Autodesk Inventor part; units mm, degrees
ref_plane "YZ Plane" through (0, 0, 0) normal (1, 0, 0) x (0, 1, 0)
ref_plane "XZ Plane" through (0, 0, 0) normal (0, 1, 0) x (-1, 0, 0)
ref_plane "XY Plane" through (0, 0, 0) normal (0, 0, 1) x (1, 0, 0)
sketch "Sketch1" plane through (0, 0, 0) normal (0, 1, 0) x (-1, 0, 0)
  line L0 (9.8554, 3.698) -> (9.8554, -5.5599)
  line L1 (0, 0) -> (-5.6892, 0)
  circle A0 centre (-2.8446, 0) radius 1.5875
  circle A1 centre (-2.8446, -12.7) radius 1.5875
  circle A2 centre (-2.8446, -25.4) radius 1.5875
  circle A3 centre (-2.8446, -38.1) radius 1.5875
  line L2 (0, 12.7) -> (-5.6892, 12.7)
  circle A4 centre (-2.8446, 12.7) radius 1.5875
  line L3 (0, 25.4) -> (-5.6892, 25.4)
  circle A5 centre (-2.8446, 25.4) radius 1.5875
  line L4 (0, 38.1) -> (-5.6892, 38.1)
  circle A6 centre (-2.8446, 38.1) radius 1.5875
  line L5 (-12.7, 0) -> (-18.3892, 0)
  circle A7 centre (-15.5446, 0) radius 1.5875
  line L6 (-25.4, 0) -> (-31.0892, 0)
  circle A8 centre (-28.2446, 0) radius 1.5875
  line L7 (-38.1, 0) -> (-43.7892, 0)
  circle A9 centre (-40.9446, 0) radius 1.5875
  line L8 (-50.8, 0) -> (-56.4892, 0)
  circle A10 centre (-53.6446, 0) radius 1.5875
  line L9 (-63.5, 0) -> (-69.1892, 0)
  circle A11 centre (-66.3446, 0) radius 1.5875
  line L10 (9.8554, 3.698) -> (9.8554, 44.45)
  line L11 (9.8554, 44.45) -> (-15.5446, 44.45)
  line L12 (-15.5446, 44.45) -> (-15.5446, 12.7)
  line L13 (-15.5446, 12.7) -> (-72.6946, 12.7)
  line L14 (-72.6946, 12.7) -> (-72.6946, -12.7)
  line L15 (-72.6946, -12.7) -> (-15.5446, -12.7)
  line L16 (-15.5446, -12.7) -> (-15.5446, -44.45)
  line L17 (-15.5446, -44.45) -> (9.8554, -44.45)
  line L18 (9.8554, -5.5599) -> (9.8554, -44.45)
  line L19 (-12.3696, 44.45) -> (-15.5446, 41.275)
  line L20 (6.6804, 44.45) -> (9.8554, 41.275)
  line L21 (9.8554, -41.275) -> (6.6804, -44.45)
  line L22 (-15.5446, -41.275) -> (-12.3696, -44.45)
  line L23 (-69.5196, 12.7) -> (-72.6946, 9.525)
  line L24 (-72.6946, -9.525) -> (-69.5196, -12.7)
  point P0 (-72.6946, 0)
  point P1 (-66.3446, 0)
  dimension "d0" = 3.175
  dimension "d1" = 12.7
  dimension "d4" = 12.7
  dimension "d11" = 12.7
  dimension "d18" = 12.7
  dimension "d23" = 25.4
  dimension "d24" = 6.35
  dimension "d25" = 12.7
  dimension "d26" = 6.35
  dimension "d27" = 25.4
extrude "Extrusion1" add sketch "Sketch1" along normal blind 3.175 contours L0 L18 L21 L17 L22 L16 L15 L24 L14 L23 L13 L12 L19 L11 L20 L10
properties part number "T-Bracket"
Part model, mm, in its own coordinate system. A direction names the side the tool comes from. Round coordinates to 2 decimals unless told otherwise and drop trailing zeros. Write each loop counter-clockwise with the first axis right and the second up, starting at its lowest first coordinate (ties: lowest second). Pieces come first, ordered by that corner, then holes.
Item 1: Drop flat-ended pins along their axis: pin 1 Ø1.9 at (x, z) = (2.84, 25.4) entering from +Y; pin 2 Ø1 at (x, y) = (50, 2) entering from -Z; pin 3 Ø1 at (y, z) = (2, 20.5) entering from +X; pin 4 Ø1 at (x, y) = (45, 2) entering from +Z. Give the stop position or say it passes through.
Results:
pin 1: passes through
pin 2: stops at z = -12.7
pin 3: stops at x = 15.54
pin 4: stops at z = 12.7
Item 2: Cut at D-D, the plane z = 0. Give the cut face in (x, y) (3 decimals), plus the area to 3 significant figures.
Results:
outline: (-9.855, 0) - (1.257, 0) - (1.257, 3.175) - (-9.855, 3.175) - close; (4.432, 0) - (13.957, 0) - (13.957, 3.175) - (4.432, 3.175) - close; (17.132, 0) - (26.657, 0) - (26.657, 3.175) - (17.132, 3.175) - close; (29.832, 0) - (39.357, 0) - (39.357, 3.175) - (29.832, 3.175) - close; (42.532, 0) - (52.057, 0) - (52.057, 3.175) - (42.532, 3.175) - close; (55.232, 0) - (64.757, 0) - (64.757, 3.175) - (55.232, 3.175) - close; (67.932, 0) - (72.695, 0) - (72.695, 3.175) - (67.932, 3.175) - close
area: 202 mm2
Item 3: Cut at C-C, the plane x = 66. Give the cut face in (y, z) (3 decimals).
Results:
outline: (0, -12.7) - (3.175, -12.7) - (3.175, -1.55) - (0, -1.55) - close; (0, 1.55) - (3.175, 1.55) - (3.175, 12.7) - (0, 12.7) - close
Item 4: Two-plate mould, pull along Z, no slides. Class faces 1 (the flat face through (23, 3.175, 1)), 2 (the cylindrical face through (42.53, 1.57, -0.07)), 3 (the flat face through (71.085, 1.565, 11.135)): +Z half, -Z half, draft (parallel to the pull), parting line (faces both ways), or undercut.
Results:
face 1: draft
face 2: undercut
face 3: +Z half
Item 5: Cut at A-A, the plane z = 25.4. Give the cut face in (x, y) (3 decimals), plus the area to 3 significant figures.
Results:
outline: (-9.855, 0) - (1.257, 0) - (1.257, 3.175) - (-9.855, 3.175) - close; (4.432, 0) - (15.545, 0) - (15.545, 3.175) - (4.432, 3.175) - close
area: 70.6 mm2
Item 6: Cut at B-B, the plane y = 2.25. Count the separate pieces of the cut face and the enclosed holes in it, plus the area to 3 significant figures.
Results:
separate pieces: 1
enclosed holes: 12
area: 3,580 mm2
Item 7: Which spindle directions (+Z, -Z, +X, -X, +Y, -Y) get a long thin tool onto all of the face, cutting with end or side? Do faces 4 (the flat face through (15.545, 2, -27)), 5 (the flat face through (15.545, 2, 27)), 6 (the flat face through (-8.29, 1.57, -42.84)). Say none if no direction does.
Results:
face 4: -Z, +X, +Y, -Y
face 5: +Z, +X, +Y, -Y
face 6: -Z, -X, +Y, -Y
Item 8: Probe L1, parallel to X at y = 1.15, z = 25.4; L2, parallel to X at y = 0.95, z = 35.5; L3, parallel to Z at x = 64, y = 3. List the from-to ranges inside material, lowest first.
Results:
L1: x = -9.86 to 1.26, 4.43 to 15.54
L2: x = -9.86 to 15.54
L3: z = -12.7 to 12.7
